Model file for the job. Use its own axes, mm. Round coordinates to 2 decimals unless told otherwise and drop trailing zeros. Order: outer loops, then holes, each group sorted by start corner. A loop starts at its lowest first (then second) coordinate and runs counter-clockwise, first axis right, second up. Notation, with made-up numbers: (65, 11) - (109, 11) arc R28 ccw to (109, 39) - close; hole circle Ø1 at (79.25, -25.75). An arc over 180 degrees is marked (long way). Answer as CSV lines item,"result". Start each with the question number.
1. Band-saw the part on A-A on x = -2.5. List the corners of the cut face in (y, z).
2. Wall check: line 1 along Z through (x, y) = (1.5, 1.2); line 2 along Y through (x, z) = (0.75, 1.35); line 3 along Y through (x, z) = (-0.75, 0.4). Give the ranges that are in metal, low to high. Write a range as [from, to].
3. Pin check, flat tip, straight feed: pin 1 Ø2 at (x, y) = (-2, 2) entering from -Z. Stop position of the tip, or through.
```python
from build123d import *

# Parameters (mm, degrees)
SKETCH1_R           = 1.75
BOSS_EXTRUDE1_DEPTH = 2.3
CUT_SWEEP2_PITCH    = 0.4


with BuildPart() as part:
    # Sketch1 → Boss-Extrude1 (new body)
    with BuildSketch(Plane.XY):
        Polygon((1.593747789, -2.746507112), (3.175418826, 0.006972516), (1.581671036, 2.753479629), (-1.593747789, 2.746507112), (-3.175418826, -0.006972516), (-1.581671036, -2.753479629), align=None)
        Circle(SKETCH1_R, mode=Mode.SUBTRACT)
    extrude(amount=BOSS_EXTRUDE1_DEPTH)

    # Cut-Sweep2: arcs per turn and ends read off the stored shape
    # Cut-Sweep2: the profile of Sketch9 screwed along a right-hand helix through 10 turns, 6 arcs to a turn; built about Z, then put on its axis
    cut_sweep2_z = Axis((0, 0, 0), (0, 0, 1))
    cut_sweep2_corners = [(0, -2.056972516, -0.5), (0, -1.606972516, -0.240192379), (0, -1.606972516, -0.759807621)]
    with BuildLine(mode=Mode.PRIVATE) as cut_sweep2_profile:
        Line(cut_sweep2_corners[0], cut_sweep2_corners[1])
        Line(cut_sweep2_corners[1], cut_sweep2_corners[2])
        Line(cut_sweep2_corners[2], cut_sweep2_corners[0])
    cut_sweep2_cap = Face(cut_sweep2_profile.wire())
    cut_sweep2_turn_angles = [0, 30, 60, 90, 120, 150, 180, 210, 240, 270, 300, 330, 360]
    cut_sweep2_turn_weights = [1, 0.8660254037844387, 1, 0.8660254037844387, 1, 0.8660254037844387, 1, 0.8660254037844387, 1, 0.8660254037844387, 1, 0.8660254037844387, 1]
    cut_sweep2_turn_rails = [Edge.make_bspline([Vector(p[0], p[1], 0).rotate(cut_sweep2_z, cut_sweep2_turn_angles[k]) / cut_sweep2_turn_weights[k] + Vector(0, 0, p[2] + CUT_SWEEP2_PITCH * cut_sweep2_turn_angles[k] / 360) for k in range(13)], [0, 0, 0, 1, 1, 2, 2, 3, 3, 4, 4, 5, 5, 6, 6, 6], 2, cut_sweep2_turn_weights) for p in cut_sweep2_corners]
    cut_sweep2_turn_sides = [Face.make_surface_from_curves(cut_sweep2_turn_rails[p[0]], cut_sweep2_turn_rails[p[1]]) for p in [(0, 1), (1, 2), (2, 0)]]
    cut_sweep2 = Plane(origin=(0, 0, 0), x_dir=(-1, 0, 0), z_dir=(0, 0, 1)) * Solid(Shell([*[p.moved(Location((0, 0, CUT_SWEEP2_PITCH * i))) for i in range(10) for p in cut_sweep2_turn_sides], cut_sweep2_cap, cut_sweep2_cap.rotate(cut_sweep2_z, 3600).moved(Location((0, 0, CUT_SWEEP2_PITCH * 3600 / 360)))]))
    add(cut_sweep2, mode=Mode.SUBTRACT)


solid = part.part
```
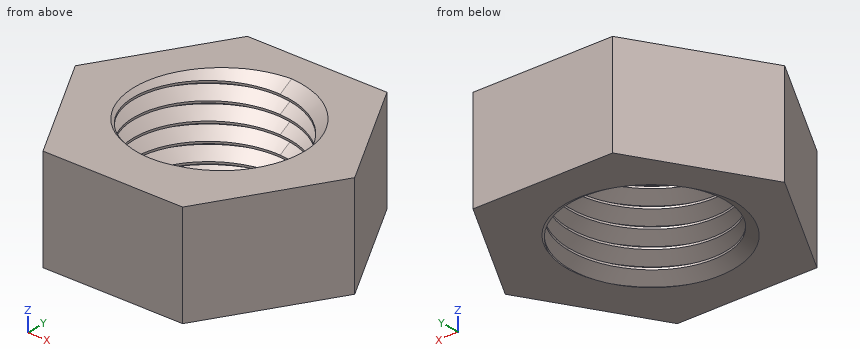
Reply:
1,outline,"(-1.17, 0) - (1.17, 0) - (1.17, 2.3) - (-1.17, 2.3) - close"
2,line 1,"z = [0, 0.16], [0.32, 0.56], [0.72, 0.96], [1.12, 1.36], [1.52, 1.76], [1.92, 2.16]"
2,line 2,"y = [-2.75, -1.87], [1.68, 2.75]"
2,line 3,"y = [-2.75, -1.78], [1.78, 2.75]"
3,pin 1,"stops at z = 0"
